Verification items for this drawing (mm, ordinates from the low corner). A direction names the side the tool comes from. Round coordinates to 2 decimals unless told otherwise and drop trailing zeros. Loops run counter-clockwise (first coordinate to the right, second up) from the corner with the lowest first, then second, coordinate; pieces in that order, holes last. Notation, with made-up numbers: (37.5, 5.25) -> (63.5, 5.25) arc R16 cw to (63.5, 27.25) -> close; hole circle Ø3 at (82, -23). An arc over 180 degrees is marked (long way). Use a Markdown table: item, result. Add a question column.
Q1. Sectioned sample at D-D, the plane x = 46. Enter the section's corners in (y, z), then the cut area to 3 significant figures.
Q2. Gauge pin test, flat ends, axial feed: P1, Ø8, axis at y = 64.5, z = 13, coming from the -X side; P2, Ø10, axis at x = 36.5, z = 33, coming from the +Y side; P3, Ø1.5, axis at x = 50.5, y = 29, coming from the +Z side. Record the tip position at first contact, or that the pin passes through.
Q3. Set-up check for the marked faces 1 and 2: record each of +Z, -Z, +X, -X, +Y, -Y from which the full face is reachable in a straight line by a thin tool's end or side.
Q4. Sectioned sample at A-A, the plane x = 18. Enter the section's corners in (y, z).
Q5. Material ranges on L1, parallel to X at y = 20, z = 2.55; L2, parallel to Z at x = 58, y = 4.2; L3, parallel to Z at x = 58, y = 2.35, recorded low to high.
Q6. Sectioned sample at B-B, the plane z = 20. Enter the section's corners in (x, y).
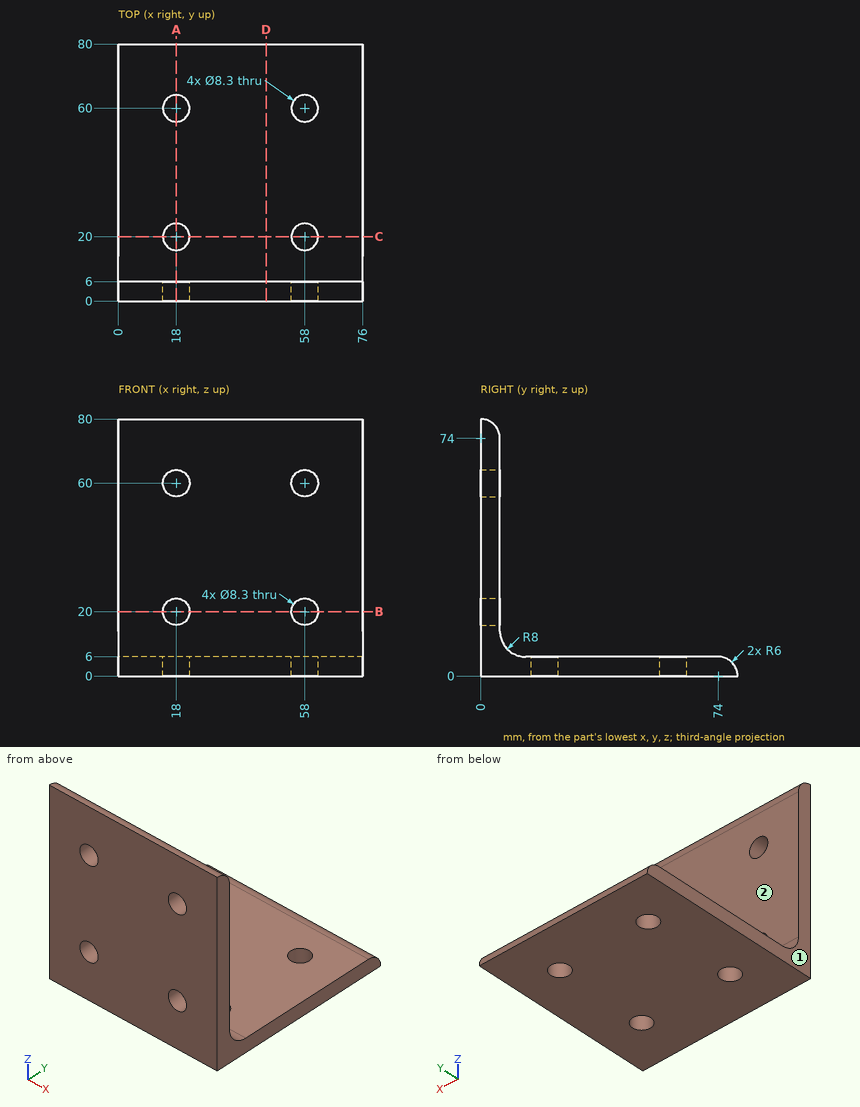
Values:
| question | item | result |
|---|---|---|
| 1 | outline | (0, 0) -> (80, 0) arc R6 ccw to (74, 6) -> (14, 6) arc R8 cw to (6, 14) -> (6, 74) arc R6 ccw to (0, 80) -> close |
| 1 | area | 922 mm^2 |
| 2 | P1 | through |
| 2 | P2 | y = 6 |
| 2 | P3 | z = 6 |
| 3 | face 1 | +Z, -Z, -X, +Y, -Y |
| 3 | face 2 | +Z, +X, -X, +Y |
| 4 | outline | (0, 0) -> (15.85, 0) -> (15.85, 6) -> (14, 6) arc R8 cw to (6, 14) -> (6, 15.85) -> (0, 15.85) -> close; (0, 24.15) -> (6, 24.15) -> (6, 55.85) -> (0, 55.85) -> close; (0, 64.15) -> (6, 64.15) -> (6, 74) arc R6 ccw to (0, 80) -> close; (24.15, 0) -> (55.85, 0) -> (55.85, 6) -> (24.15, 6) -> close; (64.15, 0) -> (80, 0) arc R6 ccw to (74, 6) -> (64.15, 6) -> close |
| 5 | L1 | 0 to 13.85, 22.15 to 53.85, 62.15 to 76 |
| 5 | L2 | 0 to 15.85, 24.15 to 55.85, 64.15 to 78.28 |
| 5 | L3 | 0 to 15.85, 24.15 to 55.85, 64.15 to 79.52 |
| 6 | outline | (0, 0) -> (13.85, 0) -> (13.85, 6) -> (0, 6) -> close; (22.15, 0) -> (53.85, 0) -> (53.85, 6) -> (22.15, 6) -> close; (62.15, 0) -> (76, 0) -> (76, 6) -> (62.15, 6) -> close |
